Geometry check sheet. Reference: the model listing, model coordinates, mm. A direction names the side the tool comes from. Give positions to 0.01 mm unless a question says otherwise; leave off trailing zeros. Write each loop counter-clockwise with the first axis right and the second up, starting at its lowest first coordinate (ties: lowest second). Pieces come first, ordered by that corner, then holes. Notation, with made-up numbers: (20.5, -29) - (35.5, -29) arc R21 cw to (35.5, 9) - close; hole circle Ø10 at (-39, 87.25). An arc over 180 degrees is marked (long way). Use a Markdown table: item, result.
```python
from build123d import *

# Parameters (mm, degrees)
CUT_EXTRUDE1_DEPTH = 5
CHAMFER1_SIZE      = 2


with BuildPart() as part:
    # Sketch1 → Revolve1 (revolve)
    with BuildSketch(Plane(origin=(0, 0, 0), x_dir=(1, 0, 0), z_dir=(0, 1, 0)), mode=Mode.PRIVATE) as revolve1_sk:
        Polygon((0, 0), (0, -370), (17.5, -370), (17.5, -350), (20, -350), (20, -140), (17.5, -140), (17.5, -120), (13, -120), (13, -70), (10, -70), (10, 0), align=None)
    revolve(revolve1_sk.sketch.rotate(Axis((0, 0, 0), (0, 0, 1)), 180), axis=Axis((0, 0, 0), (0, 0, 1)))

    # Sketch3 → Cut-Extrude1 (cut)
    with BuildSketch(Plane(origin=(-7.563219115, 20, 140), x_dir=(0, 0, -1), z_dir=(0, -1, 0))):
        with BuildLine():
            Line((-20, 13.563219115), (-60, 13.563219115))
            ThreePointArc((-60, 13.563219115), (-66, 7.563219115), (-60, 1.563219115))
            Line((-60, 1.563219115), (-20, 1.563219115))
            ThreePointArc((-20, 1.563219115), (-14, 7.563219115), (-20, 13.563219115))
        make_face()
    extrude(amount=CUT_EXTRUDE1_DEPTH, mode=Mode.SUBTRACT)

    # Chamfer1
    chamfer1_edges = [part.edges().sort_by_distance(p)[0] for p in [
        (10, 0, 0),
    ]]
    chamfer(chamfer1_edges, length=CHAMFER1_SIZE)


solid = part.part
```
1) Mould release check, pull along X, two halves, no side actions. Record for faces 1 (the flat face through (0, 18, 350)), 2 (the cylindrical face through (10.316, 7.91, 94.65)), 3 (the cylindrical face through (0, 18, 206)): pulls with the +X half, pulls with the -X half, needs draft (parallel to the pull), parting line crosses it, or undercut.
Working result:
| item | result |
|---|---|
| face 1 | needs draft |
| face 2 | parting line crosses it |
| face 3 | undercut |
2) Section check B-B on z = 228.5. Record the boundary of the cut face in (x, y).
Working result:
| item | result |
|---|---|
| outline | circle Ø40 at (0, 0) |
3) Set-up check for faces 4 (the cylindrical face through (3.794, 17.084, 359.86)), 5 (the cylindrical face through (10, 0, 36)), 6 (the flat face through (0, 15, 180)): record each of +Z, -Z, +X, -X, +Y, -Y from which the full face is reachable in a straight line by a thin tool's end or side.
Working result:
| item | result |
|---|---|
| face 4 | +Z |
| face 5 | -Z |
| face 6 | +Y |
4) Depth check by flat-ended pin: P1, Ø6, axis at x = -4.5, z = 56, coming from the +Y side; P2, Ø3.5, axis at x = -1.5, z = 174, coming from the +Y side; P3, Ø6, axis at y = -6, z = 321, coming from the +X side; P4, Ø1.5, axis at x = 12.5, y = 12.5, coming from the +Z side. Enter the tip coordinate at first touch or a pass-through.
Working result:
| item | result |
|---|---|
| P1 | stops at y = 9.89 |
| P2 | stops at y = 15 |
| P3 | stops at x = 19.77 |
| P4 | stops at z = 370 |
5) Section check A-A on x = 0. Record the boundary of the cut face in (y, z).
Working result:
| item | result |
|---|---|
| outline | (-20, 140) - (-17.5, 140) - (-17.5, 120) - (-13, 120) - (-13, 70) - (-10, 70) - (-10, 2) - (-8, 0) - (8, 0) - (10, 2) - (10, 70) - (13, 70) - (13, 120) - (17.5, 120) - (17.5, 140) - (20, 140) - (20, 154) - (15, 154) - (15, 206) - (20, 206) - (20, 350) - (17.5, 350) - (17.5, 370) - (-17.5, 370) - (-17.5, 350) - (-20, 350) - close |
6) Material ranges on L1, parallel to Z at x = -7, y = 17.5; L2, parallel to X at y = 15.5, z = 154.5; L3, parallel to Y at x = 0, z = 240, recorded low to high. Write a range as from..to.
Working result:
| item | result |
|---|---|
| L1 | z = 140..350 |
| L2 | x = -12.64..-2.4, 2.4..12.64 |
| L3 | y = -20..20 |
